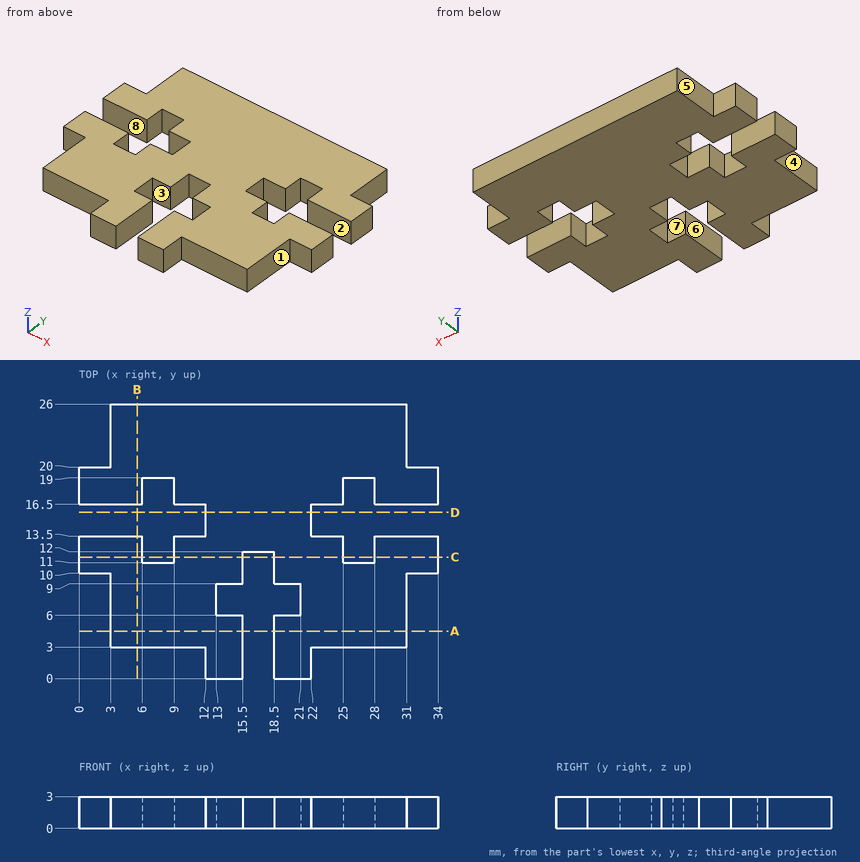
Geometry check sheet. Reference: drawing and pictorial views, mm from the part's lowest x, y, z. A direction names the side the tool comes from. Give positions to 0.01 mm unless a question says otherwise; leave off trailing zeros. Order: outer loops, then holes, each group sorted by start corner. A loop starts at its lowest first (then second) coordinate and runs counter-clockwise, first axis right, second up.
1. Section check D-D, the plane y = 15.75. Enter the section's corners in (x, z).
2. Section check A-A, the plane y = 4.5. Enter the section's corners in (x, z), and give its area (3 significant figures).
3. Gauge pin test, flat ends, axial feed: pin 1 Ø1 at (x, z) = (6, 2.5) entering from -Y; pin 2 Ø1.5 at (x, z) = (32.5, 1) entering from +Y; pin 3 Ø1.5 at (y, z) = (6.5, 1.5) entering from +X. Record the tip position at first contact, or that the pin passes through.
4. Section check C-C, the plane y = 11.5. Enter the section's corners in (x, z), and give its area (3 significant figures).
5. Section check B-B, the plane x = 5.5. Enter the section's corners in (y, z), and give its area (3 significant figures).
6. Thickness scan on L1, parallel to X at y = 12.75, z = 2.15; L2, parallel to X at y = 6.5, z = 2.35; L3, parallel to Y at x = 23, z = 2.05. Record the ranges inside material, lowest first.
7. Release check for a two-part mould opening along X. For the marked faces 5, 6, 7 and 8 record: pulls with the +X half, pulls with the -X half, needs draft (parallel to the pull), parting line crosses it, or undercut.
8. Access from +Z, -Z, +X, -X, +Y, -Y to the whole of each face (thin tool, end or side, straight path). Record for the marked faces 1, 2, 3 and 4.
Values follow:
1. outline: (12, 0) - (22, 0) - (22, 3) - (12, 3) - close
2. outline: (3, 0) - (15.5, 0) - (15.5, 3) - (3, 3) - close; (18.5, 0) - (31, 0) - (31, 3) - (18.5, 3) - close
2. area: 75.0 mm2
3. pin 1: stops at y = 3
3. pin 2: stops at y = 20
3. pin 3: stops at x = 31
4. outline: (0, 0) - (6, 0) - (6, 3) - (0, 3) - close; (9, 0) - (15.5, 0) - (15.5, 3) - (9, 3) - close; (18.5, 0) - (25, 0) - (25, 3) - (18.5, 3) - close; (28, 0) - (34, 0) - (34, 3) - (28, 3) - close
4. area: 75.0 mm2
5. outline: (3, 0) - (13.5, 0) - (13.5, 3) - (3, 3) - close; (16.5, 0) - (26, 0) - (26, 3) - (16.5, 3) - close
5. area: 60.0 mm2
6. L1: x = 0 to 6, 9 to 25, 28 to 34
6. L2: x = 3 to 13, 21 to 31
6. L3: y = 3 to 13.5, 16.5 to 26
7. face 5: pulls with the -X half
7. face 6: undercut
7. face 7: undercut
7. face 8: needs draft
8. face 1: +Z, -Z, +X, -Y
8. face 2: +Z, -Z, +X
8. face 3: +Z, -Z
8. face 4: +Z, -Z, -X, -Y
